Geometry: see drawing. Coordinates: mm, zero at the bounding-box minimum. Round coordinates to 2 decimals unless told otherwise and drop trailing zeros. Loops run counter-clockwise (first coordinate to the right, second up) from the corner with the lowest first, then second, coordinate; pieces in that order, holes last. Notation, with made-up numbers: (62, -26) -> (66, -26) arc R19 ccw to (66, 0) -> close; hole circle Ø5 at (35.5, 35). An arc over 180 degrees is marked (long way). Write item = value, one per line.
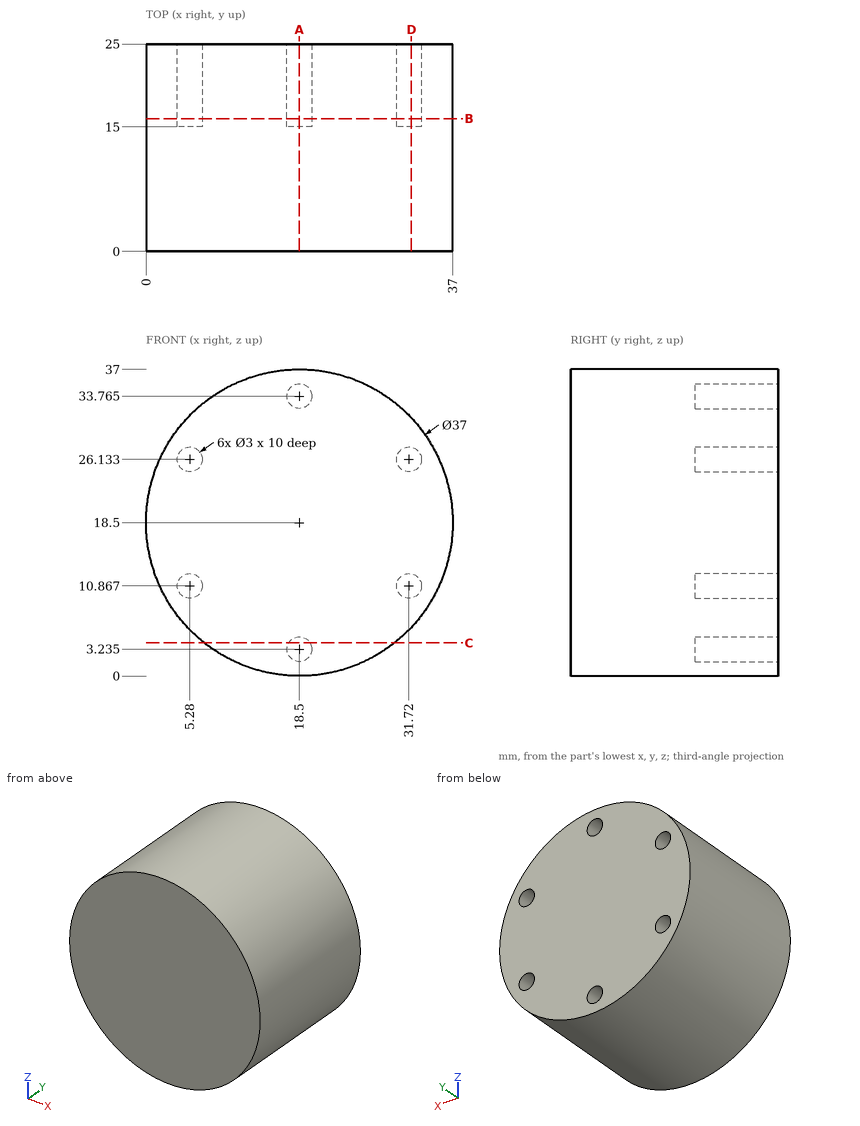
1. Section query C-C (z = 4). Return the cut outline in (x, y), then the cut area to 3 significant figures.
Evaluation:
outline = (7.01, 0) -> (29.99, 0) -> (29.99, 25) -> (19.79, 25) -> (19.79, 15) -> (17.21, 15) -> (17.21, 25) -> (7.01, 25) -> close
area = 549 mm²
2. Section query B-B (y = 16). Return the cut outline in (x, z) (1 decimal), then the cut area to 3 significant figures.
Evaluation:
outline = circle Ø37 at (18.5, 18.5); hole circle Ø3 at (5.3, 10.9); hole circle Ø3 at (5.3, 26.1); hole circle Ø3 at (18.5, 3.2); hole circle Ø3 at (18.5, 33.8); hole circle Ø3 at (31.7, 10.9); hole circle Ø3 at (31.7, 26.1)
area = 1,030 mm²
3. Line query: probe 1 along Z at (x, y) = (18.5, 21.75) (1 decimal); probe 2 along X at (y, z) = (16.5, 25) (1 decimal); probe 3 along Z at (x, y) = (18, 14.5). Output: solid intervals per line, ascending. Write a range as from..to.
Evaluation:
probe_1 = 0..1.7, 4.7..32.3, 35.3..37
probe_2 = 1.2..4.3, 6.3..30.7, 32.7..35.8
probe_3 = 0.01..36.99
4. Section query A-A (x = 18.5). Return the cut outline in (y, z) (1 decimal), then the cut area to 3 significant figures.
Evaluation:
outline = (0, 0) -> (25, 0) -> (25, 1.7) -> (15, 1.7) -> (15, 4.7) -> (25, 4.7) -> (25, 32.3) -> (15, 32.3) -> (15, 35.3) -> (25, 35.3) -> (25, 37) -> (0, 37) -> close
area = 865 mm²
5. Contact query for flat-ended pins moving along their axis: pin 1 Ø4 at (x, z) = (31.72, 26.13) entering from +Y; pin 2 Ø0.9 at (x, z) = (18.5, 34) entering from +Y; pin 3 Ø10 at (x, y) = (32.5, 11) entering from +Z; pin 4 Ø1.5 at (x, y) = (20, 19) entering from -Z (1 decimal). Output: stop coordinate, or through.
Evaluation:
pin_1 = 25
pin_2 = 15
pin_3 = 34.66
pin_4 = 0
6. Section query D-D (x = 32). Return the cut outline in (y, z).
Evaluation:
outline = (0, 5.85) -> (25, 5.85) -> (25, 9.39) -> (15, 9.39) -> (15, 12.34) -> (25, 12.34) -> (25, 24.66) -> (15, 24.66) -> (15, 27.61) -> (25, 27.61) -> (25, 31.15) -> (0, 31.15) -> close
